Could you check a few things on this model? Use its own coordinates, in mm. Face numbers are marked on the shaded views. A direction names the side the tool comes from. Coordinates: 2 decimals unless noted, no trailing zeros. Order: outer loops, then holes, each group sorted by start corner. A loop starts at its lowest first (then second) coordinate and runs counter-clockwise, first axis right, second up. Notation, with made-up numbers: (-1, 13.25) -> (18, 13.25) arc R23 ccw to (18, 33.25) -> close; hole circle Ø10 at (73, 53). An arc over 180 degrees is marked (long way). Put each result on its own line as item: value. Start each with the question number.
Q1. If we section it at C-C (x = -6.35): Please give me the cut outline in (y, z), and give its area (3 significant figures).
Q2. For the marked faces 1, 2 and 3, which set-ups out of +Z, -Z, +X, -X, +Y, -Y let a thin tool reach every point of the face, with its end or its side?
Q3. If we section it at A-A (z = -7.62): Please give me the cut outline in (x, y), and give its area (3 significant figures).
Q4. Will these pins go through, and if not, where does the flat tip stop? pin 1 (3 mm diameter, centred on y = 17, z = -12.5, fed in from +X); pin 2 (12 mm diameter, centred on x = -14.5, z = -7, fed in from +Y); pin 3 (5 mm diameter, centred on x = -27.5, y = 21, fed in from +Z).
Q5. If we section it at B-B (y = 38.5): Please give me the cut outline in (x, z), and give its area (3 significant figures).
Q6. Please list where these lines run through material, in increasing order: line 1 along X through (y, z) = (7.25, -7.62); line 2 along X through (y, z) = (37.5, -17.25); line 3 along Z through (x, y) = (-25.4, 3).
Q7. We'd pull the mould along X, two halves only. Please class the marked faces 4, 5 and 6: +X half, -X half, draft (parallel to the pull), parting line (faces both ways), or undercut.
from build123d import *

# Parameters (mm, degrees)
BOSS_EXTRUDE1_DEPTH = 31.75
CUT_EXTRUDE1_DEPTH  = 11.16
SKETCH5_R           = 1.4732
CUT_EXTRUDE2_DEPTH  = 11.16


with BuildPart() as part:
    # Sketch3 → Boss-Extrude1 (new body)
    with BuildSketch(Plane(origin=(0, 0, 0), x_dir=(0, 0, -1), z_dir=(1, 0, 0))):
        Polygon((0, 0), (25.4, 0), (25.4, 50.8), (15.24, 50.8), (15.24, 10.16), (0, 10.16), align=None)
    extrude(amount=-BOSS_EXTRUDE1_DEPTH)

    # Sketch4 → Cut-Extrude1 (cut, through all)
    with BuildSketch(Plane.XY.offset(-15.24)):
        with BuildLine():
            Line((-19.84375, 40.64), (-19.84375, 15.24))
            ThreePointArc((-19.84375, 15.24), (-15.875, 11.27125), (-11.90625, 15.24))
            Line((-11.90625, 15.24), (-11.90625, 40.64))
            ThreePointArc((-11.90625, 40.64), (-15.875, 44.60875), (-19.84375, 40.64))
        make_face()
    extrude(amount=-CUT_EXTRUDE1_DEPTH, mode=Mode.SUBTRACT)

    # Sketch5 → Cut-Extrude2 (cut, through all)
    with BuildSketch(Plane(origin=(0, 10.16, 0), x_dir=(1, 0, 0), z_dir=(0, 1, 0))):
        with Locations((-25.4, 7.62)):
            Circle(SKETCH5_R)
        with Locations((-6.35, 7.62)):
            Circle(SKETCH5_R)
    extrude(amount=-CUT_EXTRUDE2_DEPTH, mode=Mode.SUBTRACT)


solid = part.part
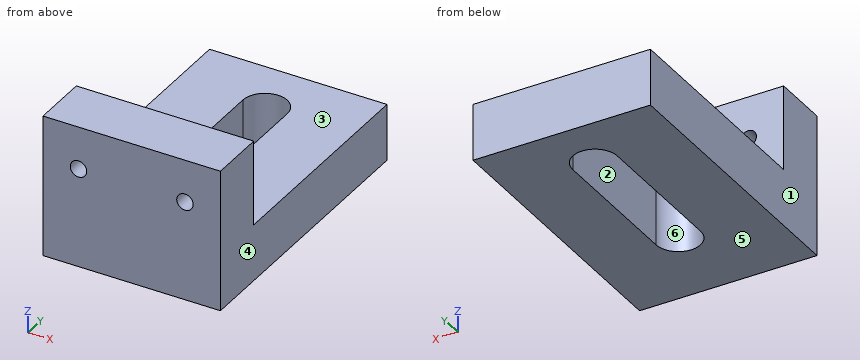
The answers:
1. outline: (0, -25.4) -> (50.8, -25.4) -> (50.8, -15.24) -> (10.16, -15.24) -> (10.16, -9.09) -> (0, -9.09) -> close; (0, -6.15) -> (10.16, -6.15) -> (10.16, 0) -> (0, 0) -> close
1. area: 641 mm^2
2. face 1: +Z, -Z, -X, +Y, -Y
2. face 2: +Z, -Z
2. face 3: +Z, +X, -X, +Y
3. outline: (-31.75, 0) -> (-26.87, 0) -> (-26.87, 10.16) -> (-31.75, 10.16) -> close; (-23.93, 0) -> (-7.82, 0) -> (-7.82, 10.16) -> (-23.93, 10.16) -> close; (-4.88, 0) -> (0, 0) -> (0, 10.16) -> (-4.88, 10.16) -> close
3. area: 263 mm^2
4. pin 1: through
4. pin 2: y = 10.16
4. pin 3: z = -15.24
5. outline: (-31.75, -25.4) -> (-19.84, -25.4) -> (-19.84, -15.24) -> (-31.75, -15.24) -> close; (-11.91, -25.4) -> (0, -25.4) -> (0, -15.24) -> (-11.91, -15.24) -> close
5. area: 242 mm^2
6. line 1: -31.75 to -26.87, -23.93 to -7.82, -4.88 to 0
6. line 2: -31.75 to -19.84, -11.91 to 0
6. line 3: -25.4 to -9.09, -6.15 to 0
7. face 4: +X half
7. face 5: draft
7. face 6: undercut
